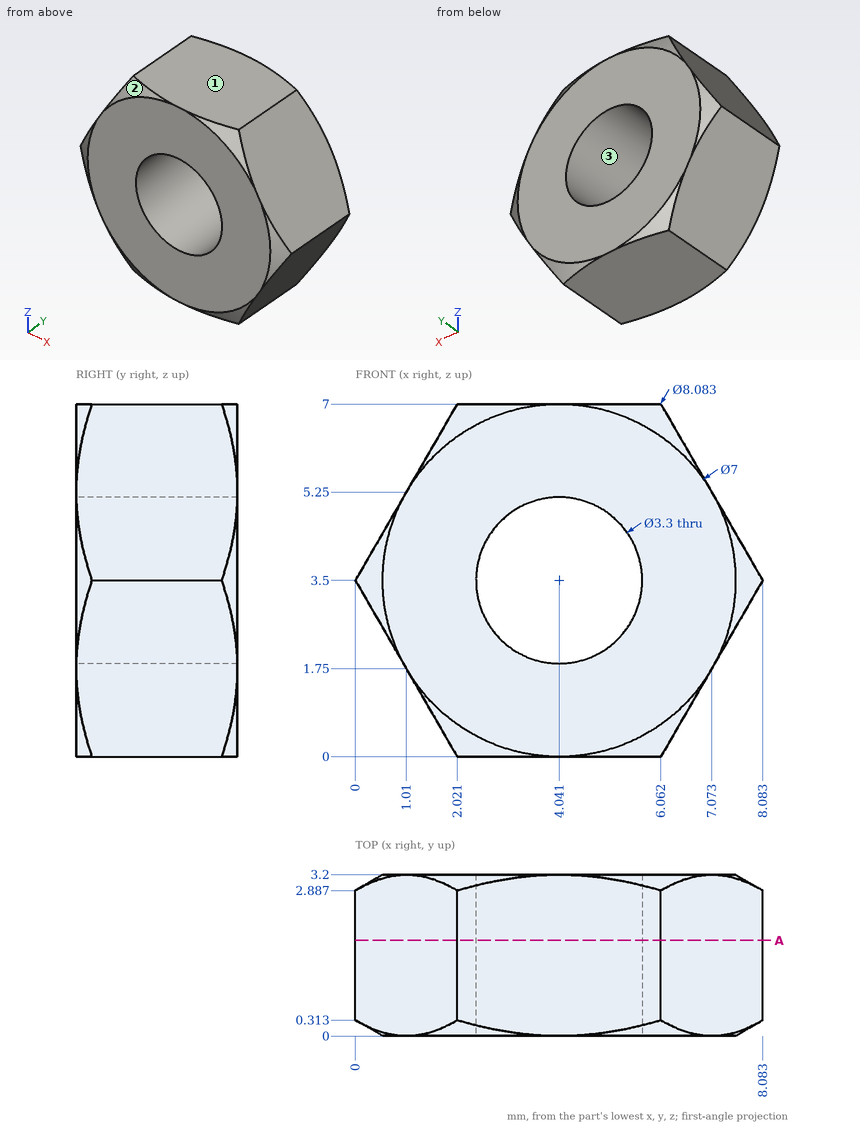
Study the drawing (mm; zero at the part's minimum x, y, z) and answer. Coordinates: 2 decimals unless noted, no trailing zeros. Loops run counter-clockwise (first coordinate to the right, second up) from the corner with the lowest first, then second, coordinate; pieces in that order, holes last. Notation, with made-up numbers: M 54,39 L 106,39 A31 cw 106,78 Z; hole C 25.5,-14 d8. An arc over 180 degrees is marked long. Answer in a Markdown table with one row per item. Add a question column.
1. The mould has two halves that part along X. Classify the marked faces 1, 2 and 3: pulls with the +X half, pulls with the -X half, needs draft (parallel to the pull), parting line crosses it, or undercut.
2. Consider L1, parallel to X at y = 1.7, z = 3.75 (1 decimal); L2, parallel to X at y = 1.75, z = 4 (1 decimal); L3, parallel to Z at x = 5.5, y = 0.5 (1 decimal). Determine where each line is inside the solid, lowest interval first.
3. Find section A-A, the plane y = 1.9. Write down the section's boundary in (x, z), then the cut area to 3 significant figures.
Reported:
| question | item | result |
|---|---|---|
| 1 | face 1 | needs draft |
| 1 | face 2 | pulls with the -X half |
| 1 | face 3 | undercut |
| 2 | L1 | x = 0.1 to 2.4, 5.7 to 7.9 |
| 2 | L2 | x = 0.3 to 2.5, 5.6 to 7.8 |
| 2 | L3 | z = 0 to 2.7, 4.3 to 7 |
| 3 | outline | M 0,3.5 L 2.02,0 L 6.06,0 L 8.08,3.5 L 6.06,7 L 2.02,7 Z; hole C 4.04,3.5 d3.3 |
| 3 | area | 33.9 mm^2 |
